```python
from build123d import *

# Parameters (mm, degrees)
SKETCH1_W           = 6.35
SKETCH1_H           = 6.35
BOSS_EXTRUDE1_DEPTH = 1.65
SKETCH2_W           = 3.81
SKETCH2_H           = 1.07
SKETCH2_H_2         = 1.02
BOSS_EXTRUDE2_DEPTH = 0.81
SKETCH3_R           = 0.38
BOSS_EXTRUDE3_DEPTH = 3.81
SKETCH4_R           = 2.675
BOSS_EXTRUDE4_DEPTH = 7.87


with BuildPart() as part:
    # Sketch1 → Boss-Extrude1 (new body)
    with BuildSketch(Plane(origin=(0, 0, 0), x_dir=(0, 0, -1), z_dir=(1, 0, 0))):
        Rectangle(SKETCH1_W, SKETCH1_H)
    extrude(amount=-BOSS_EXTRUDE1_DEPTH)

    # Sketch2 → Boss-Extrude2 (add)
    with BuildSketch(Plane(origin=(0, 0, -3.175), x_dir=(-1, 0, 0), z_dir=(0, 0, -1))):
        with Locations((-1.905, -2.64)):
            Rectangle(SKETCH2_W, SKETCH2_H)
        with Locations((-1.905, 0.135)):
            Rectangle(SKETCH2_W, SKETCH2_H_2)
    boss_extrude2 = extrude(amount=-BOSS_EXTRUDE2_DEPTH)

    # Mirror1: Boss-Extrude2 across plane
    add(boss_extrude2.mirror(Plane.XY))

    # Sketch3 → Boss-Extrude3 (add)
    with BuildSketch(Plane(origin=(0, 0, 0), x_dir=(0, 0, -1), z_dir=(1, 0, 0))):
        with Locations(Location((0, 0, 0), (0, 0, 180))):  # turned: the seam where the file's is
            Circle(SKETCH3_R)
    extrude(amount=BOSS_EXTRUDE3_DEPTH)

    # Sketch4 → Boss-Extrude4 (add)
    with BuildSketch(Plane.ZY.offset(1.65)):
        Circle(SKETCH4_R)
    extrude(amount=BOSS_EXTRUDE4_DEPTH)


solid = part.part
```
Work out the finished part from the listing and answer in its coordinate system (mm). A direction names the side the tool comes from. Coordinates: 2 decimals unless noted, no trailing zeros. Order: outer loops, then holes, each group sorted by start corner. A loop starts at its lowest first (then second) coordinate and runs counter-clockwise, first axis right, second up. Notation, with made-up numbers: (24, -31.75) - (64, -31.75) arc R11 cw to (64, -10.75) - close; hole circle Ø2 at (79, -30.5). An arc over 180 degrees is marked (long way). Answer as a JSON object with one key per item and string values.
1. Find section C-C on x = -8.25. Determine the outline of the cut face in (y, z) (3 decimals), plus the area to 3 significant figures.
Output values:
{"outline": "circle Ø5.35 at (0, 0)", "area": "22.5 mm²"}
2. Find section B-B on y = 0. Determine the outline of the cut face in (x, z) (3 decimals).
Output values:
{"outline": "(-9.52, -2.675) - (-1.65, -2.675) - (-1.65, -3.175) - (3.81, -3.175) - (3.81, -2.365) - (0, -2.365) - (0, -0.38) - (3.81, -0.38) - (3.81, 0.38) - (0, 0.38) - (0, 2.365) - (3.81, 2.365) - (3.81, 3.175) - (-1.65, 3.175) - (-1.65, 2.675) - (-9.52, 2.675) - close"}
3. A tool of negligible diameter and unlimited length cuts with its end or side. For faces 4 (the face through (-1, 3.175, 0)), 5 (the face through (-5.53, -2.61, -0.58)), 6 (the face through (2, 0, 2.365)), 7 (the face through (2, 0.645, -3)), from which of +Z, -Z, +X, -X, +Y, -Y can it reach the whole face along a straight path? Write none if from no direction.
Output values:
{"face 4": "+Z, -Z, +X, -X, +Y", "face 5": "-X", "face 6": "+X, +Y, -Y", "face 7": "+Z, -Z, +X, +Y"}
4. Each of these flat-tipped pins is pushed along its axis until it touches: P1, Ø0.9, axis at x = 2, z = 2.5, coming from the +Y side (3 decimals); P2, Ø1, axis at x = -6.5, y = -1, coming from the +Z side. Where does it stop, or does it pass through?
Output values:
{"P1": "stops at y = 0.645", "P2": "stops at z = 2.63"}
5. Find section D-D on z = -2. Determine the outline of the cut face in (x, y) (3 decimals).
Output values:
{"outline": "(-9.52, -1.776) - (-1.65, -1.776) - (-1.65, -3.175) - (0, -3.175) - (0, 3.175) - (-1.65, 3.175) - (-1.65, 1.776) - (-9.52, 1.776) - close"}
6. Find section A-A on z = 0. Determine the outline of the cut face in (x, y) (3 decimals).
Output values:
{"outline": "(-9.52, -2.675) - (-1.65, -2.675) - (-1.65, -3.175) - (0, -3.175) - (0, -0.38) - (3.81, -0.38) - (3.81, 0.38) - (0, 0.38) - (0, 3.175) - (-1.65, 3.175) - (-1.65, 2.675) - (-9.52, 2.675) - close"}
7. The mould has two halves that part along Z. Classify faces 1 (the face through (2, -2.105, 3)), 2 (the face through (0, 0, 3.175)), 3 (the face through (2, -3, -2.365)): +Z half, -Z half, draft (parallel to the pull), parting line (faces both ways), or undercut.
Output values:
{"face 1": "draft", "face 2": "+Z half", "face 3": "undercut"}
8. Consider line 1 (Z direction, x = 1, y = -2.75) (3 decimals); line 2 (X direction, y = 0, z = 2); line 3 (X direction, y = 1.5, z = -2.25). Determine where each line is inside the solid, lowest interval first.
Output values:
{"line 1": "z = -3.175 to -2.365, 2.365 to 3.175", "line 2": "x = -9.52 to 0", "line 3": "x = -1.65 to 0"}
